CAD build for the part. Positions are in the model's coordinates, mm. Give positions to 0.01 mm unless a question says otherwise; leave off trailing zeros. Loops run counter-clockwise (first coordinate to the right, second up) from the corner with the lowest first, then second, coordinate; pieces in that order, holes last.
Item 1: Saw through at C-C on y = 114. Give the cut face in (x, z), plus the area to 3 significant figures.
Item 2: Mould opens along Z. For faces 1 (the flat face through (-41.2, 250, -9.4)), 2 (the cylindrical face through (-40.06, 123.25, -12.62)), 3 (the cylindrical face through (5.598, 123.25, -42.634)) say: released by +Z, released by -Z, zero draft, split by the parting line, or undercut.
Item 3: Saw through at A-A on x = -9. Give the cut face in (y, z).
Item 4: Saw through at B-B on z = 10.5. Give the cut face in (x, y), plus the area to 3 significant figures.
Item 5: Probe probe 1 along Z at (x, y) = (0, 49.5); probe 2 along X at (y, z) = (184.5, -1); probe 3 along Z at (x, y) = (-28, 33). List the from-to ranges inside material, lowest first.
Item 6: Drop flat-ended pins along their axis: P1, Ø1, axis at y = 194, z = 25.5, coming from the -X side; P2, Ø10, axis at y = 94, z = -34, coming from the -X side; P3, Ø1.8, axis at y = 150, z = 0, coming from the +X side; P4, Ø5, axis at x = -0.5, y = 72, coming from the -Z side. Give the stop position or say it passes through.
Autodesk Inventor part; units mm, degrees
ref_plane "Work Plane2" through (0, 125, 0) normal (0, 1, 0) x (-1, 0, 0)
ref_plane "Work Plane3" through (43, 0, 0) normal (1, 0, 0) x (0, 1, 0)
ref_plane "Work Plane4" through (0, 0, 43) normal (0, 0, 1) x (1, 0, 0)
sketch "Sketch3" plane through (0, 0, 0) normal (0, 1, 0) x (-1, 0, 0)
  circle A0 centre (0, 0) radius 43
  circle A1 centre (0, 0) radius 42
  dimension "d8" = 86
  dimension "d9" = 84
extrude "Extrusion3" add sketch "Sketch3" along normal blind 250
ref_plane "Work Plane2" through (0, 125, 0) normal (0, 1, 0) x (-1, 0, 0)
sketch "Sketch4" plane through (0, 250, 0) normal (0, 1, 0) x (1, 0, 0)
  circle A0 centre (0, 42.5) radius 0.25
  point P0 (0, 0)
  dimension "d12" = 0.5
  dimension "d13" = 42.5
extrude "Extrusion4" cut sketch "Sketch4" along normal through all both and the other way through all
mirror "Mirror1" about plane through (0, 0, 0) normal (0, 0, 1) of "Extrusion4"
ref_plane "Work Plane3" through (43, 0, 0) normal (1, 0, 0) x (0, 1, 0)
sketch "Sketch5" plane through (43, 0, 0) normal (1, 0, 0) x (0, 1, 0)
  circle A0 centre (150, 0) radius 1.5
  point P0 (0, 0)
  dimension "d16" = 3
  dimension "d24" = 150
extrude "Extrusion5" cut sketch "Sketch5" against normal through all
ref_plane "Work Plane4" through (0, 0, 43) normal (0, 0, 1) x (1, 0, 0)
sketch "Sketch6" plane through (0, 0, 43) normal (0, 0, 1) x (1, 0, 0)
  circle A0 centre (-0.375, 150) radius 1.5
  point P0 (0, 0)
  dimension "d22" = 3
  dimension "d23" = 150
extrude "Extrusion6" cut sketch "Sketch6" against normal through all
properties part number "seed_holder"
Results below:
1. outline: circle Ø86 at (0, 0); hole circle Ø84 at (0, 0); hole circle Ø0.5 at (0, -42.5); hole circle Ø0.5 at (0, 42.5)
1. area: 267 mm2
2. face 1: zero draft
2. face 2: undercut
2. face 3: split by the parting line
3. outline: (0, -42.05) - (250, -42.05) - (250, -41.02) - (0, -41.02) - close; (0, 41.02) - (250, 41.02) - (250, 42.05) - (0, 42.05) - close
4. outline: (-41.7, 0) - (-40.67, 0) - (-40.67, 250) - (-41.7, 250) - close; (40.67, 0) - (41.7, 0) - (41.7, 250) - (40.67, 250) - close
4. area: 516 mm2
5. probe 1: z = -43 to -42.75, -42.25 to -42, 42 to 42.25, 42.75 to 43
5. probe 2: x = -42.99 to -41.99, 41.99 to 42.99
5. probe 3: z = -32.63 to -31.3, 31.3 to 32.63
6. P1: stops at x = -34.99
6. P2: stops at x = -31.75
6. P3: passes through
6. P4: stops at z = -43
